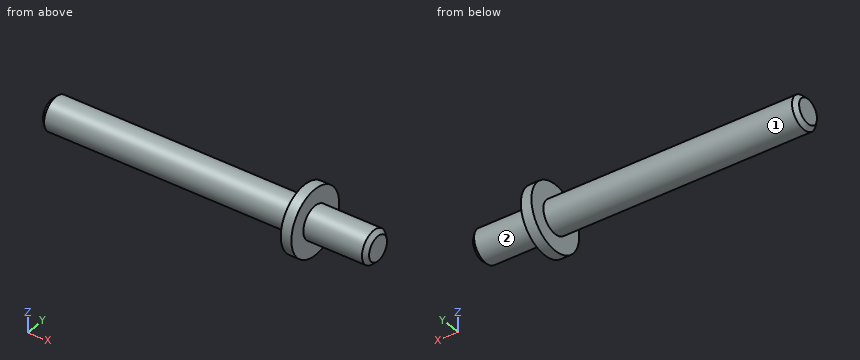
Autodesk Inventor part; units mm, degrees
ref_plane "YZ Plane" through (0, 0, 0) normal (1, 0, 0) x (0, 1, 0)
ref_plane "XZ Plane" through (0, 0, 0) normal (0, 1, 0) x (-1, 0, 0)
ref_plane "XY Plane" through (0, 0, 0) normal (0, 0, 1) x (1, 0, 0)
sketch "Sketch1" plane through (0, 0, 0) normal (0, 0, 1) x (1, 0, 0)
  line L0 (0, 0) -> (-40, 0)
  line L1 (-40, 0) -> (-40, 1.5)
  line L2 (-40, 1.5) -> (-39.5, 2)
  line L3 (-39.5, 2) -> (-9, 2)
  line L4 (-9, 2) -> (-9, 4)
  line L5 (-9, 4) -> (-7.7, 4)
  line L6 (-7.7, 4) -> (-7.7, 2)
  line L7 (-7.7, 2) -> (-0.5, 2)
  line L8 (-0.5, 2) -> (0, 1.5)
  line L9 (0, 1.5) -> (0, 0)
  dimension "d0" = 4
  dimension "d1" = 8
  dimension "d2" = 40
  dimension "d3" = 0.5
  dimension "d4" = 45
  dimension "d5" = 45
  dimension "d6" = 0.5
  dimension "d7" = 1.3
  dimension "d8" = 7.7
revolve "Revolution1" add sketch "Sketch1" angle 360 about axis through (0, 0, 0) along (-1, 0, 0)
properties part number "18102021-002-05" material "Stainless Steel"
The listing builds one solid part. Answer for the finished solid, in the listing's coordinates (mm). Face numbers are marked on the shaded views. A direction names the side the tool comes from. Give positions to 0.01 mm unless a question says otherwise; leave off trailing zeros. Write each loop counter-clockwise with the first axis right and the second up, starting at its lowest first coordinate (ties: lowest second). Pieces come first, ordered by that corner, then holes.
Item 1: Find the intervals of material crossed by line 1 along X through (y, z) = (-2.75, -2); line 2 along Y through (x, z) = (-36, 0); line 3 along Z through (x, y) = (-8.5, -2.75), in increasing order.
Item 2: Section D-D, the plane z = 3.25 is taken. Write down the section's boundary in (x, y), plus the area to 3 significant figures.
Item 3: Section A-A, the plane z = 0 is taken. Write down the section's boundary in (x, y), plus the area to 3 significant figures.
Item 4: Which of the six approach directions +Z, -Z, +X, -X, +Y, -Y give full straight-line access (tool end or side, diameter ignored) to the marked faces 1 and 2?
Item 5: Flat-ended cylindrical pins translate along their axes: P1, Ø4, axis at x = -35.5, y = 2, coming from the +Z side; P2, Ø2, axis at y = -3, z = -2.5, coming from the -X side; P3, Ø1.5, axis at x = -7.5, z = -1.5, coming from the -Y side. Find the tip coordinate at first contact, or state that the pin passes through.
Item 6: Section C-C, the plane x = -19 is taken. Write down the section's boundary in (y, z).
Completed:
1. line 1: x = -9 to -7.7
1. line 2: y = -2 to 2
1. line 3: z = -2.9 to 2.9
2. outline: (-9, -2.33) - (-7.7, -2.33) - (-7.7, 2.33) - (-9, 2.33) - close
2. area: 6.06 mm2
3. outline: (-40, -1.5) - (-39.5, -2) - (-9, -2) - (-9, -4) - (-7.7, -4) - (-7.7, -2) - (-0.5, -2) - (0, -1.5) - (0, 1.5) - (-0.5, 2) - (-7.7, 2) - (-7.7, 4) - (-9, 4) - (-9, 2) - (-39.5, 2) - (-40, 1.5) - close
3. area: 165 mm2
4. face 1: -X
4. face 2: +X
5. P1: stops at z = 2
5. P2: stops at x = -9
5. P3: stops at y = -3.92
6. outline: circle Ø4 at (0, 0)
